Build history of the part. All positions in model axes, mm. Face numbers are marked on the shaded views. A direction names the side the tool comes from. Round coordinates to 2 decimals unless told otherwise and drop trailing zeros. Write each loop counter-clockwise with the first axis right and the second up, starting at its lowest first coordinate (ties: lowest second). Pieces come first, ordered by that corner, then holes. Notation, with made-up numbers: (46, 84.25) -> (71, 84.25) arc R29 cw to (71, 110.25) -> close; hole circle Ø2 at (-21, -26.5). An arc over 180 degrees is marked (long way). One line per question, with ' | ' between items.
Autodesk Inventor part; units mm, degrees
ref_plane "YZ Plane" through (0, 0, 0) normal (1, 0, 0) x (0, 1, 0)
ref_plane "XZ Plane" through (0, 0, 0) normal (0, 1, 0) x (-1, 0, 0)
ref_plane "XY Plane" through (0, 0, 0) normal (0, 0, 1) x (1, 0, 0)
sketch "Sketch1" plane through (0, 0, 0) normal (0, 0, 1) x (1, 0, 0)
  circle A0 centre (0, 0) radius 27.5
  dimension "d0" = 55
extrude "Extrusion1" add sketch "Sketch1" along normal blind 80
sketch "Sketch2" plane through (0, 0, 80) normal (0, 0, 1) x (1, 0, 0)
  circle A0 centre (0, 0) radius 27.5
  line L0 (-22.5, -15.8114) -> (22.5, -15.8114)
  dimension "d5" = 45
extrude "Extrusion2" cut sketch "Sketch2" against normal blind 80 contours L0 A0 picked at (-6.0353, -17.4405)
sketch "Sketch3" plane through (-22.5, -15.8114, 80) normal (0, -1, 0) x (1, 0, 0)
  line L0 (43, -70) -> (2, -70)
  line L1 (2, -70) -> (2, -29)
  line L2 (2, -29) -> (43, -29)
  line L3 (43, -29) -> (43, -70)
  line L4 (0, -80) -> (0, 0)
  line L5 (45, 0) -> (45, -80)
  line L6 (0, 0) -> (45, 0)
  line L7 (45, -80) -> (0, -80)
  point P0 (22.5, -80)
  dimension "d16" = 41
  dimension "d17" = 41
  dimension "d18" = 45
  dimension "d19" = 2
  dimension "d20" = 29
extrude "Extrusion3" cut sketch "Sketch3" against normal blind 1.5 contours L0 L1 L2 L3
sketch "Sketch4" plane through (0, 0, 0) normal (0, 0, -1) x (-1, 0, 0)
  arc A0 (22.5, -15.8114) -> (-22.5, -15.8114) centre (0, 0) ccw
  circle A1 centre (0, 0) radius 25
  line L0 (21.4678, -12.8114) -> (-21.4678, -12.8114)
  line L1 (-22.5, -15.8114) -> (22.5, -15.8114)
  dimension "d12" = 50
  dimension "d13" = 3
extrude "Extrusion4" cut sketch "Sketch4" against normal blind 77 contours L0 A1
sketch "Sketch5" plane through (-22.5, -14.3114, 80) normal (0, -1, 0) x (1, 0, 0)
  circle A0 centre (22.5, -50.1203) radius 18
  point P0 (22.5, -80)
  dimension "d25" = 36
extrude "Extrusion5" cut sketch "Sketch5" against normal blind 31
hole "Hole1" at (-17.5, -14.3114, 48) direction (0, 1, 0) diameter 3 depth 8
hole "Hole2" at (17.5, -14.3114, 48) direction (0, 1, 0) diameter 3 depth 8
hole "Hole3" at (-17.5, -14.3114, 13) direction (0, 1, 0) diameter 3 depth 8
hole "Hole4" at (17.5, -14.3114, 13) direction (0, 1, 0) diameter 3 depth 8
properties part number "speaker_body"
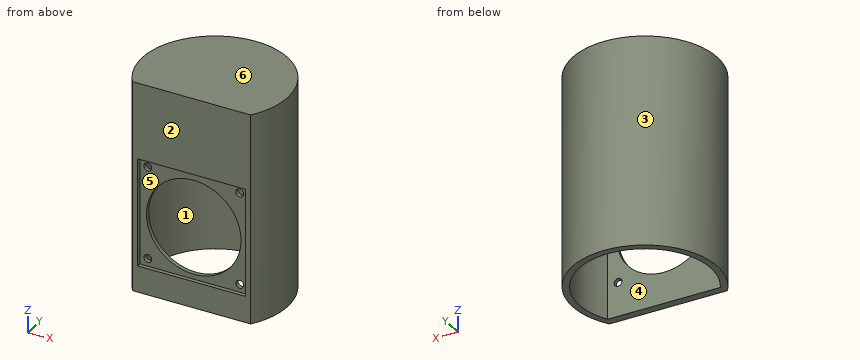
(1) Mould opens along Y. For the marked faces 1, 2, 3 and 4 say: pulls with the +Y half, pulls with the -Y half, needs draft (parallel to the pull), parting line crosses it, or undercut.
Calculated:
face 1: undercut | face 2: pulls with the -Y half | face 3: parting line crosses it | face 4: undercut
(2) 3-axis set-ups, long thin cutter, end or side, ignore diameter. For the marked faces 5 and 6: which of +Z, -Z, +X, -X, +Y, -Y reach the whole face in a straight line?
Calculated:
face 5: -Y | face 6: +Z, +X, -X, +Y, -Y
(3) Slice it at C-C (y = 0). Write the cut outline in (x, z), then the cut area to 3 significant figures.
Calculated:
outline: (-27.5, 0) -> (-25, 0) -> (-25, 77) -> (25, 77) -> (25, 0) -> (27.5, 0) -> (27.5, 80) -> (-27.5, 80) -> close | area: 550 mm2
(4) Drop flat-ended pins along their axis: pin 1 (12.5 mm diameter, centred on x = 4, z = 29.5, fed in from -Y); pin 2 (10 mm diameter, centred on y = 22, z = 34.5, fed in from +X); pin 3 (5 mm diameter, centred on x = -17.5, z = 13, fed in from +Y). Give the stop position or say it passes through.
Calculated:
pin 1: y = 22.8 | pin 2: x = 21.62 | pin 3: y = 23.05
(5) Slice it at A-A (x = 0). Write the cut outline in (y, z).
Calculated:
outline: (-15.81, 0) -> (-12.81, 0) -> (-12.81, 11.88) -> (-14.31, 11.88) -> (-14.31, 10) -> (-15.81, 10) -> close; (-15.81, 51) -> (-14.31, 51) -> (-14.31, 47.88) -> (-12.81, 47.88) -> (-12.81, 77) -> (25, 77) -> (25, 0) -> (27.5, 0) -> (27.5, 80) -> (-15.81, 80) -> close
(6) Slice it at D-D (x = 14.5). Write the cut outline in (y, z), then the cut area to 3 significant figures.
Calculated:
outline: (-15.81, 0) -> (-12.81, 0) -> (-12.81, 19.21) -> (-14.31, 19.21) -> (-14.31, 10) -> (-15.81, 10) -> close; (-15.81, 51) -> (-14.31, 51) -> (-14.31, 40.55) -> (-12.81, 40.55) -> (-12.81, 77) -> (20.37, 77) -> (20.37, 0) -> (23.37, 0) -> (23.37, 80) -> (-15.81, 80) -> close | area: 486 mm2
(7) Wall check: line 1 (Z direction, x = 22, y = 8.5); line 2 (Z direction, x = 0, y = -13.3); line 3 (X direction, y = 23, z = 30). Give the ranges that are in metal, low to high. Write a range as from..to.
Calculated:
line 1: 77..80 | line 2: 0..11.88, 47.88..80 | line 3: -15.07..-9.8, 9.8..15.07
(8) Slice it at B-B (z = 13). Write the cut outline in (x, y), then the cut area to 3 significant figures.
Calculated:
outline: (-22.5, -15.81) -> (-20.5, -15.81) -> (-20.5, -14.31) -> (-19, -14.31) -> (-19, -12.81) -> (-21.47, -12.81) arc R25 cw (long way) to (21.47, -12.81) -> (19, -12.81) -> (19, -14.31) -> (20.5, -14.31) -> (20.5, -15.81) -> (22.5, -15.81) arc R27.5 ccw (long way) to start; (-16, -14.31) -> (-6.25, -14.31) -> (-6.25, -12.81) -> (-16, -12.81) -> close; (6.25, -14.31) -> (16, -14.31) -> (16, -12.81) -> (6.25, -12.81) -> close | area: 325 mm2
